Can you work these out from the model? Positions are in its coordinate system, mm. Face numbers are marked on the shaded views. Give positions to 0.01 mm unless a question says otherwise; leave off trailing zeros. Order: outer loops, then holes, each group sorted by start corner. A loop starts at its lowest first (then second) coordinate and runs counter-clockwise, first axis right, second up. Notation, with made-up numbers: M -1.75,-23.5 L 7.25,-23.5 A18 ccw 7.25,-12.5 Z; hole C -4.75,-24.5 d4. An arc over 180 degrees is marked long. Use a Markdown table: item, result. Add a question column.
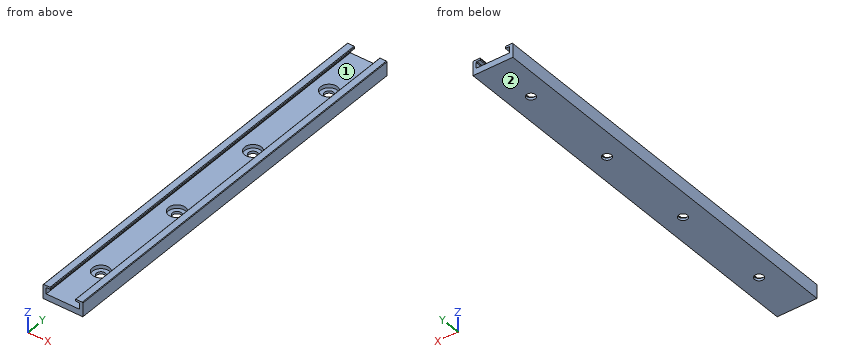
Autodesk Inventor part; units mm, degrees
ref_plane "YZ Plane" through (0, 0, 0) normal (1, 0, 0) x (0, 1, 0)
ref_plane "XZ Plane" through (0, 0, 0) normal (0, 1, 0) x (-1, 0, 0)
ref_plane "XY Plane" through (0, 0, 0) normal (0, 0, 1) x (1, 0, 0)
sketch "スケッチ1" plane through (0, 0, 0) normal (0, 1, 0) x (-1, 0, 0)
  line L0 (-10, 0) -> (10, 0)
  line L1 (10, 0) -> (10, 7.2)
  line L2 (10, 7.2) -> (6.2, 7.2)
  line L3 (8.4, 3) -> (-8.4, 3)
  line L4 (-6.2, 7.2) -> (-10, 7.2)
  line L5 (-10, 7.2) -> (-10, 0)
  line L6 (6.2, 7.2) -> (6.2, 6.2)
  line L7 (6.2, 6.2) -> (8.4, 6.2)
  line L8 (8.4, 6.2) -> (8.4, 3)
  line L9 (-6.2, 7.2) -> (-6.2, 6.2)
  line L10 (-6.2, 6.2) -> (-8.4, 6.2)
  line L11 (-8.4, 6.2) -> (-8.4, 3)
  point P0 (0, 0)
  point P1 (0, 0)
  point P2 (0, 3)
  dimension "d0" = 20
  dimension "d1" = 7.2
  dimension "d2" = 3
  dimension "d3" = 12.4
  dimension "d4" = 1
  dimension "d22" = 16.8
extrude "押し出し1" add sketch "スケッチ1" along normal blind 200
chamfer "面取り1" distance 0.3 angle 45 7 edges at (-10, 100, 7.2) (-6.2, 100, 7.2) (6.2, 100, 6.2) (6.2, 100, 7.2) (10, 100, 7.2) (8.4, 100, 6.2) (-8.4, 100, 6.2)
sketch "スケッチ2" plane through (-8.4, 0, 3) normal (0, 0, 1) x (1, 0, 0)
  line L0 (0, 0) -> (16.8, 0) construction
  point P0 (8.4, 0)
  point P1 (8.4, 25)
  point P2 (8.4, 0)
  dimension "d11" = 25
hole "穴1" at (0, 25, 3) direction (0, 0, -1) diameter 4.5 end through all counterbore diameter 8.5 counterbore depth 1.8
pattern_linear "矩形状パターン1" count 10 spacing 50 along (0, 1, 0) of "穴1"
equation "\"d6\" = Length"
equation "\"Length\" = 200"
properties part number "MRS20-200" material "アルミニウム 6061"
1. If we section it at B-B, the plane z = 4.75: List the corners of the cut face in (x, y) for me.
2. If we section it at D-D, the plane x = 0: State how many separate pieces and enclosed holes the cut face has, then the cut area to 3 significant figures.
3. If we section it at A-A, the plane y = 75: List the corners of the cut face in (x, z) for me.
4. We'd pull the mould along Z, two halves only. Please class the marked faces 1 and 2: +Z half, -Z half, draft (parallel to the pull), parting line (faces both ways), or undercut.
5. I need wall thicknesses on L1, parallel to Y at x = 0, z = 1.8; L2, parallel to Y at x = 0, z = 0.4; L3, parallel to X at y = 108, z = 4. Which ranges of each line are inside material? Lowest first, please. Write a range as [from, to].
6. If we section it at C-C, the plane y = 34: List the corners of the cut face in (x, z) for me.
7. Will these pins go through, and if not, where does the flat tip stop? pin 1 (4 mm diameter, centred on x = -1.5, y = 177, fed in from +Z); pin 2 (3.5 mm diameter, centred on x = 0, y = 125, fed in from +Z); pin 3 (5 mm diameter, centred on x = 0, y = 125, fed in from +Z).
Geometry results:
| question | item | result |
|---|---|---|
| 1 | outline | M -10,0 L -8.4,0 L -8.4,200 L -10,200 Z; M 8.4,0 L 10,0 L 10,200 L 8.4,200 Z |
| 2 | separate pieces | 5 |
| 2 | enclosed holes | 0 |
| 2 | area | 517 mm^2 |
| 3 | outline | M -10,0 L -2.25,0 L -2.25,1.2 L -4.25,1.2 L -4.25,3 L -8.4,3 L -8.4,5.9 L -8.1,6.2 L -6.2,6.2 L -6.2,6.9 L -6.5,7.2 L -9.7,7.2 L -10,6.9 Z; M 2.25,0 L 10,0 L 10,6.9 L 9.7,7.2 L 6.5,7.2 L 6.2,6.9 L 6.2,6.5 L 6.5,6.2 L 8.1,6.2 L 8.4,5.9 L 8.4,3 L 4.25,3 L 4.25,1.2 L 2.25,1.2 Z |
| 4 | face 1 | undercut |
| 4 | face 2 | -Z half |
| 5 | L1 | y = [0, 20.75], [29.25, 70.75], [79.25, 120.75], [129.25, 170.75], [179.25, 200] |
| 5 | L2 | y = [0, 22.75], [27.25, 72.75], [77.25, 122.75], [127.25, 172.75], [177.25, 200] |
| 5 | L3 | x = [-10, -8.4], [8.4, 10] |
| 6 | outline | M -10,0 L 10,0 L 10,6.9 L 9.7,7.2 L 6.5,7.2 L 6.2,6.9 L 6.2,6.5 L 6.5,6.2 L 8.1,6.2 L 8.4,5.9 L 8.4,3 L -8.4,3 L -8.4,5.9 L -8.1,6.2 L -6.2,6.2 L -6.2,6.9 L -6.5,7.2 L -9.7,7.2 L -10,6.9 Z |
| 7 | pin 1 | stops at z = 3 |
| 7 | pin 2 | passes through |
| 7 | pin 3 | stops at z = 1.2 |
